Verification items for the finished model (mm, model axes). Give positions to 0.01 mm unless a question says otherwise; leave off trailing zeros. Return JSON: item names as keys, results as strings. Group by question number.
(1) Thickness scan on line 1 along X through (y, z) = (-19.5, 2.2); line 2 along Y through (x, z) = (28, 2.9); line 3 along Y through (x, z) = (88, 1.65). Record the ranges inside material, lowest first.
(2) Cross-section at A-A on z = 0.5. State how many separate pieces and enclosed holes the cut face has, then the cut area to 3 significant figures.
(3) Depth check by flat-ended pin: pin 1 Ø1.6 at (x, z) = (30.5, 1.5) entering from -Y; pin 2 Ø1 at (y, z) = (-5.5, 0.5) entering from +X; pin 3 Ø0.8 at (x, z) = (1.5, 1.5) entering from +Y. Enter the tip coordinate at first touch or a pass-through.
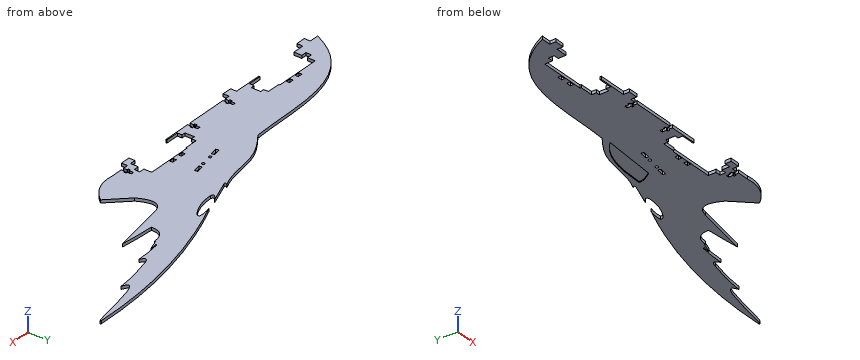
from build123d import *

# Parameters (mm, degrees)
BOSS_EXTRUDE1_DEPTH = 3.175
SKETCH3_W           = 10
SKETCH3_H           = 6.35
BOSS_EXTRUDE2_DEPTH = 3.175
CUT_EXTRUDE1_DEPTH  = 1
CUT_EXTRUDE2_DEPTH  = 309.914260869
SKETCH7_W           = 5
SKETCH7_H           = 3.175
CUT_EXTRUDE3_DEPTH  = 309.914260869
SKETCH8_R           = 1.5
CUT_EXTRUDE4_DEPTH  = 309.914260869


with BuildPart() as part:
    # Sketch2 → Boss-Extrude1 (new body)
    with BuildSketch(Plane.XY):
        with BuildLine():
            Line((-171.469047232, -34.076589663), (107.072734851, -34.076589663))
            add(Edge.make_bspline(
                [(107.072734851, -34.076589663), (128.968224532, -36.583015685), (142.892082906, -18.715522774)],
                knots=[0, 0, 0, 1, 1, 1], degree=2))
            Line((142.892082906, -18.715522774), (122.99960361, 1.8225486))
            add(Edge.make_bspline(
                [(129.812103759, 28.346921979), (110.367502019, 24.835662341), (122.99960361, 1.8225486)],
                knots=[0, 0, 0, 1, 1, 1], degree=2))
            Line((129.812103759, 28.346921979), (185.982982819, 38.244685161))
            add(Edge.make_bspline(
                [(150.588622768, 41.132714976), (168.332466646, 40.241827569), (185.982982819, 38.244685161)],
                knots=[0, 0, 0, 1, 1, 1], degree=2))
            add(Edge.make_bspline(
                [(166.211544782, 56.600045126), (150.111599454, 56.448151942), (150.588622768, 41.132714976)],
                knots=[0, 0, 0, 1, 1, 1], degree=2))
            Line((166.211544782, 56.600045126), (166.232711914, 57.669663084))
            Line((166.232711914, 57.669663084), (177.243348067, 61.403308501))
            add(Edge.make_bspline(
                [(177.243348067, 61.403308501), (173.339529375, 61.796609349), (169.627135034, 60.610840144)],
                knots=[0, 0, 0, 1, 1, 1], degree=2))
            add(Edge.make_bspline(
                [(169.627135034, 60.610840144), (169.762853876, 62.544945332), (172.402329475, 62.156522878)],
                knots=[0, 0, 0, 1, 1, 1], degree=2))
            add(Edge.make_bspline(
                [(172.402329475, 62.156522878), (184.617311888, 64.041519989), (197.029812567, 63.947302758)],
                knots=[0, 0, 0, 1, 1, 1], degree=2))
            add(Edge.make_bspline(
                [(197.029812567, 63.947302758), (187.73474396, 69.069639789), (198.964387884, 71.402059066)],
                knots=[0, 0, 0, 1, 1, 1], degree=2))
            add(Edge.make_bspline(
                [(198.964387884, 71.402059066), (219.003547299, 76.786528717), (239.76459105, 78.329887141)],
                knots=[0, 0, 0, 1, 1, 1], degree=2))
            add(Edge.make_bspline(
                [(291.780939868, 98.47138823), (303.090852198, 95.717715254), (210.844028254, 88.026417155), (239.76459105, 78.329887141)],
                knots=[0, 0, 0, 0, 1, 1, 1, 1], degree=3))
            add(Edge.make_bspline(
                [(291.780939868, 98.47138823), (190.608851514, 100.539390251), (97.737935683, 60.775941524)],
                knots=[0, 0, 0, 1, 1, 1], degree=2))
            add(Edge.make_bspline(
                [(97.737935683, 60.775941524), (104.92881908, 63.001143493), (112.379572637, 62.156522878)],
                knots=[0, 0, 0, 1, 1, 1], degree=2))
            add(Edge.make_bspline(
                [(112.379572637, 62.156522878), (112.730110756, 59.051830939), (109.55036868, 57.311722682)],
                knots=[0, 0, 0, 1, 1, 1], degree=2))
            add(Edge.make_bspline(
                [(109.55036868, 57.311722682), (96.530025853, 49.246897899), (81.058579137, 49.55282081)],
                knots=[0, 0, 0, 1, 1, 1], degree=2))
            add(Edge.make_bspline(
                [(81.058579137, 49.55282081), (75.642299748, 50.628036984), (83.696612356, 55.998318906)],
                knots=[0, 0, 0, 1, 1, 1], degree=2))
            Line((83.696612356, 55.998318906), (60.023408157, 47.198036308))
            add(Edge.make_bspline(
                [(60.023408157, 47.198036308), (56.150260782, 46.24516321), (59.12376331, 49.613311176)],
                knots=[0, 0, 0, 1, 1, 1], degree=2))
            add(Edge.make_bspline(
                [(59.12376331, 49.613311176), (44.292473838, 41.921501166), (13.209344651, 43.405332099), (-7.707186428, 29.993825045), (-18.106560521, 22.301338951)],
                knots=[0, 0, 0, 0, 0.606338938, 1, 1, 1, 1], degree=3))
            add(Edge.make_bspline(
                [(-18.106560521, 22.301338951), (-73.30010729, 18.178725753), (-142.381543794, 32.928841514), (-171.469047232, -34.076589663)],
                knots=[0, 0, 0, 0, 1, 1, 1, 1], degree=3))
        make_face()
    extrude(amount=BOSS_EXTRUDE1_DEPTH)

    # Sketch3 → Boss-Extrude2 (add)
    with BuildSketch(Plane.XY.offset(3.175)):
        with Locations((-156.469047232, -37.251589663)):
            Rectangle(SKETCH3_W, SKETCH3_H)
        with Locations((-56.469047232, -37.251589663)):
            Rectangle(SKETCH3_W, SKETCH3_H)
        with Locations((81.530952768, -37.251589663)):
            Rectangle(SKETCH3_W, SKETCH3_H)
    extrude(amount=-BOSS_EXTRUDE2_DEPTH)

    # Sketch4 → Cut-Extrude1 (cut)
    with BuildSketch(Plane.XY):
        with BuildLine():
            Line((-8.735344321, 21.076667257), (49.27249451, 25.443679203))
            add(Edge.make_bspline(
                [(55.435775055, 40.720887474), (56.710717132, 34.955549426), (51.7521577, 29.95185464), (49.27249451, 25.443679203)],
                knots=[0, 0, 0, 0, 1, 1, 1, 1], degree=3))
            add(Edge.make_bspline(
                [(55.435775055, 40.720887474), (33.054612951, 40.360145045), (7.874054379, 39.272954497), (-8.735344321, 21.076667257)],
                knots=[0, 0, 0, 0, 1, 1, 1, 1], degree=3))
        make_face()
    extrude(amount=CUT_EXTRUDE1_DEPTH, mode=Mode.SUBTRACT)

    # Sketch5 → Cut-Extrude2 (cut, through all)
    with BuildSketch(Plane.XY.offset(3.175)):
        Polygon((-45.969047232, -34.076589663), (-42.969047232, -34.076589663), (-42.969047232, -30.276589663), (-41.419047232, -30.276589663), (-41.419047232, -27.876589663), (-42.969047232, -27.876589663), (-42.969047232, -23.426589663), (-45.969047232, -23.426589663), (-45.969047232, -27.876589663), (-47.519047232, -27.876589663), (-47.519047232, -30.276589663), (-45.969047232, -30.276589663), align=None)
        Polygon((2.030952768, -30.276589663), (2.030952768, -34.076589663), (5.030952768, -34.076589663), (5.030952768, -30.276589663), (6.580952768, -30.276589663), (6.580952768, -27.876589663), (5.030952768, -27.876589663), (5.030952768, -23.426589663), (2.030952768, -23.426589663), (2.030952768, -27.876589663), (0.480952768, -27.876589663), (0.480952768, -30.276589663), align=None)
        Polygon((92.030952768, -30.276589663), (92.030952768, -34.076589663), (95.030952768, -34.076589663), (95.030952768, -30.276589663), (96.580952768, -30.276589663), (96.580952768, -27.876589663), (95.030952768, -27.876589663), (95.030952768, -23.426589663), (92.030952768, -23.426589663), (92.030952768, -27.876589663), (90.480952768, -27.876589663), (90.480952768, -30.276589663), align=None)
    extrude(amount=-CUT_EXTRUDE2_DEPTH, mode=Mode.SUBTRACT)

    # Sketch7 → Cut-Extrude3 (cut, through all)
    with BuildSketch(Plane.XY.offset(3.175)):
        Polygon((-91.469047232, -32.876589663), (-77.469047232, -32.876589663), (-77.469047232, -27.876589663), (-73.469047232, -27.876589663), (-73.469047232, -17.876589663), (-77.469047232, -17.876589663), (-77.469047232, -12.876589663), (-91.469047232, -12.876589663), (-91.469047232, -11.676589663), (-139.469047232, -11.676589663), (-139.469047232, -19.876589663), (-144.969047232, -19.876589663), (-144.969047232, -25.876589663), (-139.469047232, -25.876589663), (-139.469047232, -34.076589663), (-91.469047232, -34.076589663), align=None)
        Polygon((20.530952768, -27.876589663), (20.530952768, -32.876589663), (34.530952768, -32.876589663), (34.530952768, -34.076589663), (82.530952768, -34.076589663), (82.530952768, -25.876589663), (88.030952768, -25.876589663), (88.030952768, -19.876589663), (82.530952768, -19.876589663), (82.530952768, -11.676589663), (34.530952768, -11.676589663), (34.530952768, -12.876589663), (20.530952768, -12.876589663), (20.530952768, -17.876589663), (16.530952768, -17.876589663), (16.530952768, -27.876589663), align=None)
        with Locations((-113.769047232, -9.149089663)):
            Rectangle(SKETCH7_W, SKETCH7_H)
        with Locations((-101.769047232, -9.149089663)):
            Rectangle(SKETCH7_W, SKETCH7_H)
        with Locations((44.830952768, -9.149089663)):
            Rectangle(SKETCH7_W, SKETCH7_H)
        with Locations((56.830952768, -9.149089663)):
            Rectangle(SKETCH7_W, SKETCH7_H)
    extrude(amount=-CUT_EXTRUDE3_DEPTH, mode=Mode.SUBTRACT)

    # Sketch8 → Cut-Extrude4 (cut, through all)
    with BuildSketch(Plane(origin=(0, 0, 0), x_dir=(-1, 0, 0), z_dir=(0, 0, -1))):
        with Locations((-33.483463602, 11.904038041)):
            Circle(SKETCH8_R)
        with Locations(Location((-45.301156639, 13.987816173, 0), (0, 0, 180))):
            Circle(SKETCH8_R)
        Polygon((-20.405296331, 11.209994039), (-20.956629295, 8.083229423), (-28.835091319, 9.472414844), (-28.283758355, 12.59917946), align=None)
        Polygon((-49.949528922, 16.419439369), (-50.500861886, 13.292674753), (-58.37932391, 14.681860174), (-57.827990946, 17.80862479), align=None)
    extrude(amount=-CUT_EXTRUDE4_DEPTH, mode=Mode.SUBTRACT)


solid = part.part
Verdict:
{
 "1": {"line 1": "-163.74 to -139.47, -73.47 to 16.53, 82.53 to 142.27", "line 2": "-34.08 to -32.88, -12.88 to 9.33, 12.55 to 41.75", "line 3": "-34.08 to -25.88, -19.88 to 49.85"},
 "2": {"separate pieces": "1", "enclosed holes": "9", "area": "18,800 mm²"},
 "3": {"pin 1": "y = -34.08", "pin 2": "x = 130.58", "pin 3": "y = 34.98"}
}
